Verification items for the finished model (mm, model axes). Face numbers are marked on the shaded views. A direction names the side the tool comes from. Coordinates: 2 decimals unless noted, no trailing zeros. Write each loop counter-clockwise with the first axis right and the second up, starting at its lowest first coordinate (ties: lowest second). Pieces come first, ordered by that corner, then holes. Notation, with made-up numbers: (-21.75, 27) -> (10.25, 27) arc R28 cw to (10.25, 56) -> close; hole circle Ø8 at (37, 78.25). An arc over 180 degrees is marked (long way). Use CSV: the item, a comma, the result in double quotes.
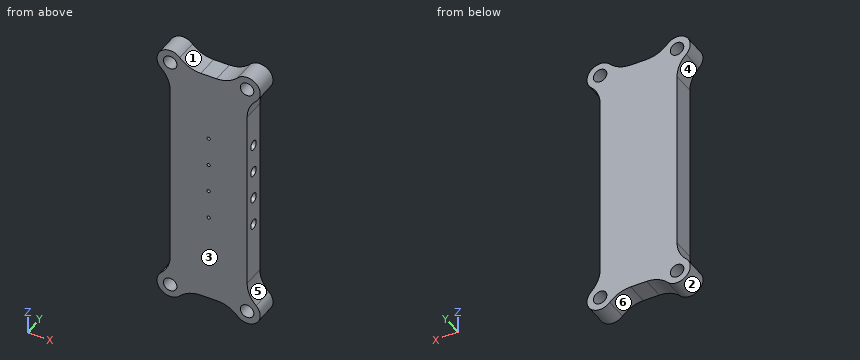
```python
from build123d import *

# Parameters (mm, degrees)
F0_R     = 2.1
F1_DEPTH = 7
F2_R     = 0.5
F3_DEPTH = 4
F4_R     = 1.5
F5_DEPTH = 13


with BuildPart() as f1:
    # F0 (on Front) → F1 (new body)
    with BuildSketch(Plane.XZ):
        with BuildLine():
            ThreePointArc((2.979207, -11.709161), (5.958651, -9.626508), (9.518929, -8.892367))
            Line((9.518929, -8.892367), (14.481071, -8.892367))
            ThreePointArc((14.481071, -8.892367), (18.041349, -9.626508), (21.020793, -11.709161))
            ThreePointArc((21.020793, -11.709161), (26.899138, -11.791505), (26.816794, -5.913161))
            ThreePointArc((26.816794, -5.913161), (24.734141, -2.933716), (24, 0.626561))
            Line((24, 0.626561), (24, 57.588704))
            ThreePointArc((24, 57.588704), (24.734141, 61.148981), (26.816794, 64.128426))
            ThreePointArc((26.816794, 64.128426), (26.899138, 70.006771), (21.020793, 69.924427))
            ThreePointArc((21.020793, 69.924427), (18.041349, 67.841774), (14.481071, 67.107633))
            Line((14.481071, 67.107633), (9.578815, 67.107633))
            ThreePointArc((9.578815, 67.107633), (5.999651, 67.849934), (3.010891, 69.954391))
            ThreePointArc((3.010891, 69.954391), (-2.873666, 70.057006), (-2.797957, 64.172041))
            ThreePointArc((-2.797957, 64.172041), (-0.715304, 61.192596), (0.018837, 57.632319))
            Line((0.018837, 57.632319), (0.018837, 0.644336))
            ThreePointArc((0.018837, 0.644336), (-0.718827, -2.92411), (-2.810898, -5.907597))
            ThreePointArc((-2.810898, -5.907597), (-2.902002, -11.788638), (2.979207, -11.709161))
        make_face()
        with Locations((0, -8.892367)):
            Circle(F0_R, mode=Mode.SUBTRACT)
        with Locations((24, -8.892367)):
            Circle(F0_R, mode=Mode.SUBTRACT)
        with Locations((0.018837, 67.151248)):
            Circle(F0_R, mode=Mode.SUBTRACT)
        with Locations((24, 67.107633)):
            Circle(F0_R, mode=Mode.SUBTRACT)
    extrude(amount=F1_DEPTH)

    # F2 (on face) → F3 (cut)
    with BuildSketch(Plane.XZ.offset(7)):
        with Locations((12.018837, 45.629388)):
            Circle(F2_R)
        with Locations((12.018837, 36.629373)):
            Circle(F2_R)
        with Locations((12.018837, 27.629358)):
            Circle(F2_R)
        with Locations((12.018837, 18.629343)):
            Circle(F2_R)
    extrude(amount=-F3_DEPTH, mode=Mode.SUBTRACT)

    # F4 (on face) → F5 (cut)
    with BuildSketch(Plane.YZ.offset(24)):
        with Locations((-3.5, 45.607704)):
            Circle(F4_R)
        with Locations((-3.5, 36.607704)):
            Circle(F4_R)
        with Locations((-3.5, 27.607704)):
            Circle(F4_R)
        with Locations((-3.5, 18.607704)):
            Circle(F4_R)
    extrude(amount=-F5_DEPTH, mode=Mode.SUBTRACT)


solid = f1.part
```
1) Gauge pin test, flat ends, axial feed: pin 1 (3 mm diameter, centred on x = 8.5, z = 5.5, fed in from +Y); pin 2 (4 mm diameter, centred on y = -3.5, z = 45.61, fed in from -X); pin 3 (2 mm diameter, centred on x = 10, y = -1, fed in from -Z); pin 4 (2 mm diameter, centred on y = -5, z = 23.5, fed in from +X). Record the tip position at first contact, or that the pin passes through.
Return value:
pin 1,"y = 0"
pin 2,"x = 0.02"
pin 3,"z = -8.91"
pin 4,"x = 24"
2) Mould release check, pull along Z, two halves, no side actions. Record for the marked faces 1, 2 and 3: released by +Z, released by -Z, zero draft, split by the parting line, or undercut.
Return value:
face 1,"released by +Z"
face 2,"undercut"
face 3,"zero draft"
3) Cross-section at D-D (x = 5.5). Record the boundary of the cut face in (y, z).
Return value:
outline,"(-7, -9.84) -> (0, -9.84) -> (0, 68.08) -> (-7, 68.08) -> close"
4) Cross-section at B-B (z = 30). Record the boundary of the cut face in (x, y), plus the area to 3 significant figures.
Return value:
outline,"(0.02, -7) -> (24, -7) -> (24, 0) -> (0.02, 0) -> close"
area,"168 mm2"
5) Cross-section at A-A (x = 18.5). Record the boundary of the cut face in (y, z), plus the area to 3 significant figures.
Return value:
outline,"(-7, -9.84) -> (0, -9.84) -> (0, 68.05) -> (-7, 68.05) -> close; hole circle Ø3 at (-3.5, 18.61); hole circle Ø3 at (-3.5, 27.61); hole circle Ø3 at (-3.5, 36.61); hole circle Ø3 at (-3.5, 45.61)"
area,"517 mm2"
6) Scan lines: L1, parallel to X at y = -3.25, z = 67; L2, parallel to Z at x = 18, y = -4; L3, parallel to Z at x = 18, y = -4.75. Record each from-to range of solid material in increasing order.
Return value:
L1,"-4.08 to -2.08, 2.11 to 21.9, 26.1 to 28.1"
L2,"-9.61 to 17.19, 20.02 to 26.19, 29.02 to 35.19, 38.02 to 44.19, 47.02 to 67.82"
L3,"-9.61 to 17.78, 19.44 to 26.78, 28.44 to 35.78, 37.44 to 44.78, 46.44 to 67.82"
7) Set-up check for the marked faces 4, 5 and 6: record each of +Z, -Z, +X, -X, +Y, -Y from which the full face is reachable in a straight line by a thin tool's end or side.
Return value:
face 4,"-X, +Y, -Y"
face 5,"+X, +Y, -Y"
face 6,"-Z, +Y, -Y"
8) Cross-section at C-C (y = -3.5). Give the number of separate pieces and of enclosed holes in the cut face, plus the area to 3 significant figures.
Return value:
separate pieces,"1"
enclosed holes,"4"
area,"1,800 mm2"
